For this review, take the finished solid that the model builds, in its own axes (mm). A direction names the side the tool comes from. Round coordinates to 2 decimals unless told otherwise and drop trailing zeros. Order: outer loops, then holes, each group sorted by start corner. A loop starts at its lowest first (then second) coordinate and runs counter-clockwise, first axis right, second up. Notation, with made-up numbers: M 29,-32.75 L 63,-32.75 A29 cw 63,-2.75 Z; hole C 62.25,15 d2. An arc over 180 degrees is marked long. Answer in a Markdown table with one row per item. Add a question column.
```python
from build123d import *

# Parameters (mm, degrees)
SKETCH2_R               = 2.5
SKETCH2_R_2             = 0.6
SKETCH2_R_3             = 1
BOSS_EXTRUDE2_DEPTH     = 2
BOSS_EXTRUDE3_DEPTH     = 3.2
BOSS_EXTRUDE4_OUTLINE_R = 0.6
BOSS_EXTRUDE4_DEPTH     = 1.5
SKETCH5_R               = 1
CUT_EXTRUDE1_DEPTH      = 46.971757445


# Read off the part's stored shape, not the designer's step: Boss-Extrude4
with BuildPart() as part:
    # Sketch2 → Boss-Extrude2 (new body)
    # profile 1 of 3: a face of its own
    with BuildSketch(Plane(origin=(0, 0, 0), x_dir=(1, 0, 0), z_dir=(0, 1, 0))):
        with BuildLine():
            ThreePointArc((2.5, 0), (2.144922946, -1.284252917), (1.180555556, -2.203698841))
            ThreePointArc((1.180555556, -2.203698841), (21.25, 2.833420868), (41.319444444, -2.203698841))
            ThreePointArc((41.319444444, -2.203698841), (40.296301159, 1.180555556), (43.680555556, 2.203698841))
            ThreePointArc((43.680555556, 2.203698841), (21.25, 7.833420868), (-1.180555556, 2.203698841))
            ThreePointArc((-1.180555556, 2.203698841), (1.284252917, 2.144922946), (2.5, 0))
        make_face()
    # profile 2 of 3: a face of its own
    with BuildSketch(Plane(origin=(0, 0, 0), x_dir=(1, 0, 0), z_dir=(0, 1, 0))):
        with Locations((42.5, 0)):
            Circle(SKETCH2_R)
        with Locations(Location((42.5, 0, 0), (0, 0, 270))):
            Circle(SKETCH2_R_2, mode=Mode.SUBTRACT)
    # profile 3 of 3: a face of its own
    with BuildSketch(Plane(origin=(0, 0, 0), x_dir=(1, 0, 0), z_dir=(0, 1, 0))):
        Circle(SKETCH2_R)
        with Locations(Location((0, 0, 0), (0, 0, 270))):
            Circle(SKETCH2_R_3, mode=Mode.SUBTRACT)
    extrude(amount=BOSS_EXTRUDE2_DEPTH)

    # Sketch3 → Boss-Extrude3 (add)
    with BuildSketch(Plane(origin=(0, 2, 0), x_dir=(1, 0, 0), z_dir=(0, 1, 0))):
        with BuildLine():
            ThreePointArc((41.798567685, 3.158721406), (21.784485497, 7.830413671), (1.670343314, 3.610285866))
            Line((1.670343314, 3.610285866), (9.157651663, 1.076826613))
            ThreePointArc((9.157651663, 1.076826613), (22.148316133, 2.823926021), (35.053533161, 0.529346934))
            Line((35.053533161, 0.529346934), (41.798567685, 3.158721406))
        make_face()
    extrude(amount=BOSS_EXTRUDE3_DEPTH)

    # Boss-Extrude4 outline → Boss-Extrude4 (add)
    with BuildSketch(Plane(origin=(0, 2, 0), x_dir=(1, 0, 0), z_dir=(0, 1, 0))):
        with BuildLine():
            Line((41.798567685, 3.158721406), (35.053533161, 0.529346934))
            ThreePointArc((35.053533161, 0.529346934), (38.241528411, -0.710989517), (41.319444444, -2.203698841))
            ThreePointArc((41.319444444, -2.203698841), (44.703698841, -1.180555556), (43.680555556, 2.203698841))
            ThreePointArc((43.680555556, 2.203698841), (42.744866263, 2.691663565), (41.798567685, 3.158721406))
        make_face()
        with Locations((42.5, 0)):
            Circle(BOSS_EXTRUDE4_OUTLINE_R, mode=Mode.SUBTRACT)
    extrude(amount=BOSS_EXTRUDE4_DEPTH)

    # Sketch5 → Cut-Extrude1 (cut, through all)
    with BuildSketch(Plane(origin=(0, 5.2, 0), x_dir=(1, 0, 0), z_dir=(0, 1, 0))):
        with Locations(Location((12.25, 4.424236239, 0), (0, 0, 270))):
            Circle(SKETCH5_R)
        with Locations(Location((30.25, 4.424236239, 0), (0, 0, 270))):
            Circle(SKETCH5_R)
    extrude(amount=-CUT_EXTRUDE1_DEPTH, mode=Mode.SUBTRACT)


solid = part.part
```
1. For faces 4 (the flat face through (21, 0, -4)), 5 (the flat face through (41, 3.5, 0)), list the 3-axis set-ups (+Z, -Z, +X, -X, +Y, -Y) from which the entire face can be reached by the end or side of a thin tool; tool diameter is ignored.
2. Consider section C-C on z = -1.5. Write out the cut boundary in (x, y).
3. Clearance check with flat-ended pins moving along their axes: pin 1 Ø3 at (x, y) = (28.5, 1) entering from -Z; pin 2 Ø1.7 at (x, z) = (41, -0.5) entering from +Y; pin 3 Ø1 at (x, y) = (13, 1) entering from -Z. State where each tip first meets the part, or that it passes through.
4. Consider section D-D on x = 2.5. Write out the cut boundary in (y, z).
5. Consider section B-B on y = 2.45. Write out the cut boundary in (x, z), plus the area to 3 significant figures.
6. Consider section A-A on x = 12.25. Write out the cut boundary in (y, z), plus the area to 3 significant figures.
7. To check wall thickness, follow probe 1 along X at (y, z) = (3.15, -4.25); probe 2 along Y at (x, z) = (2.5, -2.25); probe 3 along Z at (x, y) = (42.5, 1.5). State the ranges of each line that lie inside material, in increasing order. Write a range as [from, to].
8. The part is to be moulded in two halves that separate along X. For faces 1 (the cylindrical face through (11.274, 2.636, -4.641)), 2 (the flat face through (2, 2, -1)), 3 (the flat face through (5.36, 3.58, -2.36)), say which applies: pulls with the +X half, pulls with the -X half, needs draft (parallel to the pull), parting line crosses it, or undercut.
Solved:
| question | item | result |
|---|---|---|
| 1 | face 4 | +Z, -Z, +X, -X, -Y |
| 1 | face 5 | +Z, +X, +Y |
| 2 | outline | M -2,0 L 10.69,0 L 10.69,5.2 L 7.91,5.2 L 7.91,2 L -2,2 Z; M 31.81,0 L 44.5,0 L 44.5,3.5 L 37.54,3.5 L 37.54,5.2 L 31.81,5.2 Z |
| 3 | pin 1 | stops at z = -7.48 |
| 3 | pin 2 | stops at y = 3.5 |
| 3 | pin 3 | stops at z = -7.2 |
| 4 | outline | M 0,-3.98 L 5.2,-3.98 L 5.2,-3.33 L 2,-3.33 L 2,1.53 L 0,1.53 Z |
| 5 | outline | M 1.67,-3.61 A47.5 ccw 41.8,-3.16 A47.5 ccw 43.68,-2.2 A2.5 ccw 41.32,2.2 A42.5 cw 9.16,-1.08 Z; hole C 12.25,-4.42 d2; hole C 30.25,-4.42 d2; hole C 42.5,0 d1.2 |
| 5 | area | 195 mm^2 |
| 6 | outline | M 0,-6.97 L 5.2,-6.97 L 5.2,-5.42 L 0,-5.42 Z; M 0,-3.42 L 5.2,-3.42 L 5.2,-1.87 L 0,-1.87 Z |
| 6 | area | 16.1 mm^2 |
| 7 | probe 1 | x = [3.15, 11.27], [13.23, 29.27], [31.23, 39.35] |
| 7 | probe 2 | y = [0, 2] |
| 7 | probe 3 | z = [-2.82, -0.6], [0.6, 2.5] |
| 8 | face 1 | undercut |
| 8 | face 2 | needs draft |
| 8 | face 3 | pulls with the -X half |
